Input: dimensioned drawing with shaded views. Units: mm. Origin: part minimum x, y, z. Coordinates: 2 decimals unless noted, no trailing zeros. Loops run counter-clockwise (first coordinate to the right, second up) from the corner with the lowest first, then second, coordinate; pieces in that order, holes last. Notation, with made-up numbers: (-3, 50) - (13, 50) arc R18 cw to (13, 60) - close; hole circle Ø1 at (53, -18). An arc over 180 degrees is marked (long way). Write item = value, one per line. Start each with the question number.
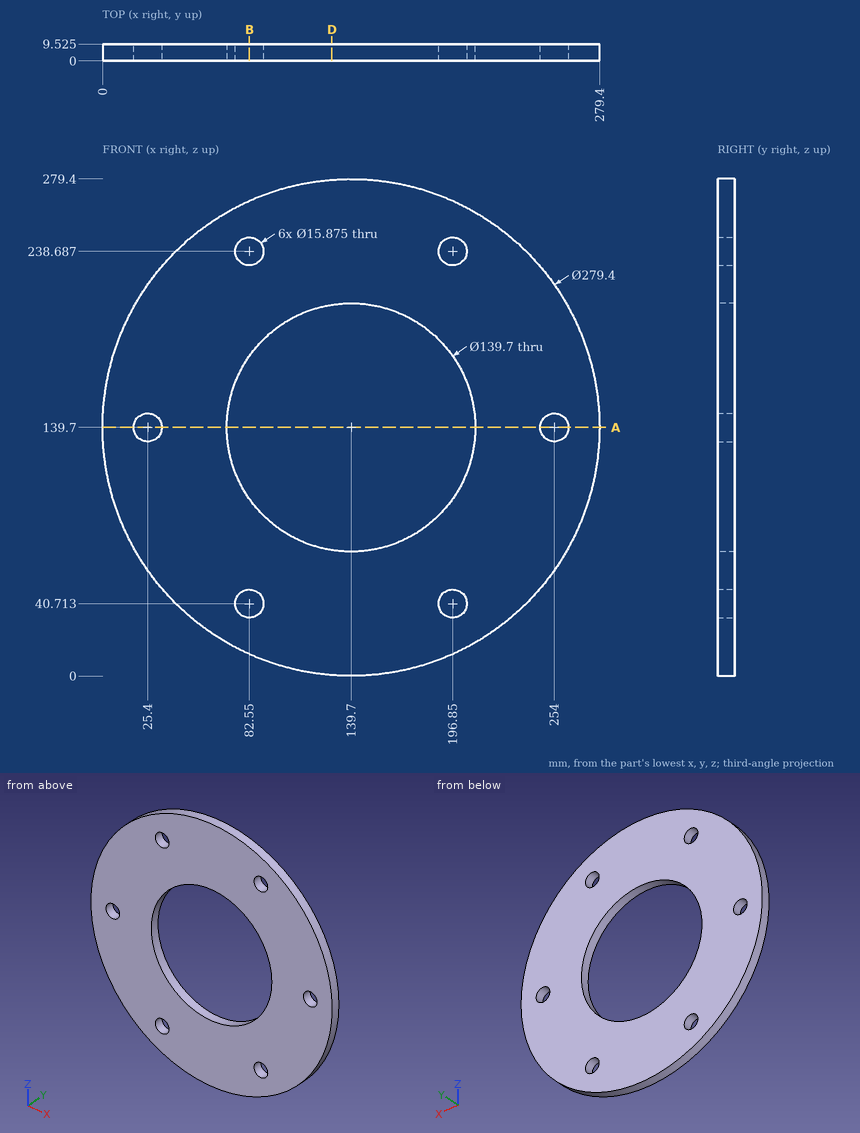
Item 1: Ray query, line 1 (X direction, y = 8.75, z = 35); line 2 (Z direction, x = 139.7, y = 5.75); line 3 (X direction, y = 3.75, z = 137.5) (1 decimal). Return the intervals inside material, ascending.
Item 2: Cut plane B-B on x = 82.55. Return loops of the section in (y, z) (1 decimal).
Item 3: Pin query (flat end, axial travel): pin 1 (20.5 mm diameter, centred on x = 196.85, z = 238.69, fed in from -Y); pin 2 (2 mm diameter, centred on x = 222, y = 7.5, fed in from +Z); pin 3 (14.5 mm diameter, centred on x = 196.85, z = 40.71, fed in from -Y); pin 4 (5 mm diameter, centred on y = 5, z = 107.5, fed in from -X). Return the tip coordinate at first contact, or that it passes through.
Item 4: Cut plane A-A on z = 139.7. State how many separate pieces and enclosed holes the cut face has, plus the area to 3 significant figures.
Item 5: Cut plane D-D on x = 129. Return loops of the section in (y, z) (1 decimal).
Recorded:
q1.line_1 = 47.21 to 77.04, 88.06 to 191.34, 202.36 to 232.19
q1.line_2 = 0 to 69.85, 209.55 to 279.4
q1.line_3 = 0 to 17.8, 33 to 69.9, 209.5 to 246.4, 261.6 to 279.4
q2.outline = (0, 12.2) - (9.5, 12.2) - (9.5, 32.8) - (0, 32.8) - close; (0, 48.7) - (9.5, 48.7) - (9.5, 99.5) - (0, 99.5) - close; (0, 179.9) - (9.5, 179.9) - (9.5, 230.7) - (0, 230.7) - close; (0, 246.6) - (9.5, 246.6) - (9.5, 267.2) - (0, 267.2) - close
q3.pin_1 = 0
q3.pin_2 = 253.31
q3.pin_3 = through
q3.pin_4 = 3.19
q4.separate_pieces = 4
q4.enclosed_holes = 0
q4.area = 1,030 mm²
q5.outline = (0, 0.4) - (9.5, 0.4) - (9.5, 70.7) - (0, 70.7) - close; (0, 208.7) - (9.5, 208.7) - (9.5, 279) - (0, 279) - close
